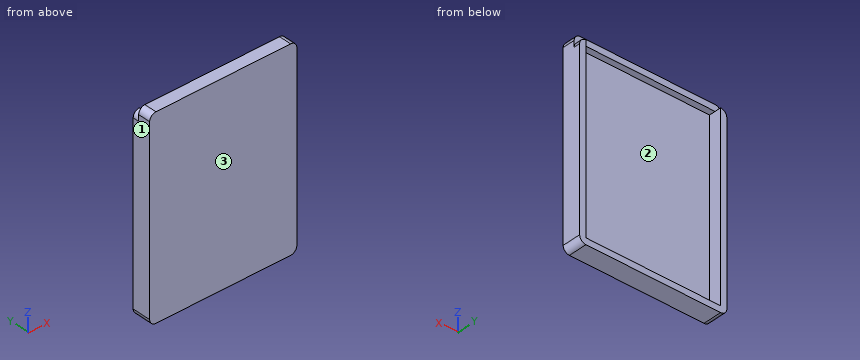
Autodesk Inventor part; units mm, degrees
ref_plane "YZ Plane" through (0, 0, 0) normal (1, 0, 0) x (0, 1, 0)
ref_plane "XZ Plane" through (0, 0, 0) normal (0, 1, 0) x (-1, 0, 0)
ref_plane "XY Plane" through (0, 0, 0) normal (0, 0, 1) x (1, 0, 0)
sketch "Sketch1" plane through (0, 0, 0) normal (0, 1, 0) x (-1, 0, 0)
  line L0 (-23.55, -31) -> (23.55, -31)
  line L1 (23.55, -31) -> (23.55, 31)
  line L2 (23.55, 31) -> (-23.55, 31)
  line L3 (-23.55, 31) -> (-23.55, -31)
  line L4 (-23.55, -31) -> (23.55, 31) construction
  line L5 (23.55, -31) -> (-23.55, 31) construction
  point P0 (0, 0)
  dimension "d0" = 47.1
  dimension "d1" = 62
extrude "Extrusion1" add sketch "Sketch1" along normal blind 2
sketch "Sketch2" plane through (0, 2, 0) normal (0, 1, 0) x (1, 0, 0)
  line L0 (-23.55, 31) -> (-23.55, -31)
  line L1 (23.55, -31) -> (23.55, 31)
  line L2 (-23.55, -31) -> (23.55, -31)
  line L3 (23.55, -31) -> (23.55, 31)
  line L4 (23.55, 31) -> (-23.55, 31)
  line L5 (-23.55, 31) -> (-23.55, -31)
  line L6 (-21.55, -29) -> (21.55, -29)
  line L7 (21.55, -29) -> (21.55, 29)
  line L8 (21.55, 29) -> (-21.55, 29)
  line L9 (-21.55, 29) -> (-21.55, -29)
  point P0 (0, 0)
  dimension "d4" = 2
  dimension "d5" = 2
  dimension "d6" = 2
  dimension "d7" = 2
extrude "Extrusion2" add sketch "Sketch2" along normal blind 2
sketch "Sketch3" plane through (0, 4, 0) normal (0, 1, 0) x (1, 0, 0)
  line L0 (-23.55, 31) -> (-23.55, -31)
  line L1 (23.55, 31) -> (-23.55, 31)
  line L2 (-23.55, 31) -> (-23.55, -29)
  line L3 (23.55, -29) -> (23.55, 31)
  line L4 (21.55, 29) -> (21.55, -29)
  line L5 (-21.55, -29) -> (-21.55, 29)
  line L6 (21.55, 29) -> (-21.55, 29)
  line L7 (-21.55, 29) -> (-21.55, -29)
  line L8 (-21.55, -29) -> (21.55, -29)
  line L9 (21.55, -29) -> (21.55, 29)
  line L10 (-21.55, -29) -> (-23.55, -29)
  line L11 (21.55, -29) -> (23.55, -29)
  line L12 (23.55, -31) -> (23.55, 31)
  line L13 (-23.55, -31) -> (23.55, -31)
  point P0 (0, 0)
extrude "Extrusion3" add sketch "Sketch3" along normal blind 2 contours L1 L3 L11 L4 L6 L5 L10 L0
fillet "Fillet1" radius 2 6 edges at (23.55, 2, 31) (23.55, 3, -31) (-23.55, 3, -31) (-23.55, 5, 29) (23.55, 5, 29) (-23.55, 2, 31)
properties part number "esp_shield_holder"
Input: part model. Units: mm. Frame: model coordinates. Face numbers are marked on the shaded views. Round coordinates to 2 decimals unless told otherwise and drop trailing zeros. Loops run counter-clockwise (first coordinate to the right, second up) from the corner with the lowest first, then second, coordinate; pieces in that order, holes last. Notation, with made-up numbers: (-21, 21.5) -> (21, 21.5) arc R19 ccw to (21, 57.5) -> close; hole circle Ø9 at (-33, -17.75). An arc over 180 degrees is marked (long way). Answer as a JSON object with one key per item and string values. Group by question number.
1) Ray query, L1, parallel to X at y = 4.5, z = -15; L2, parallel to Z at x = 19, y = 3.1; L3, parallel to Z at x = 16.5, y = 5.35. Return the intervals inside material, ascending.
2) Pin query (flat end, axial travel): pin 1 (10 mm diameter, centred on x = -9, z = 5.5, fed in from +Y); pin 2 (4.5 mm diameter, centred on x = 2.5, z = 28.5, fed in from +Y). Return the tip coordinate at first contact, or that it passes through.
3) Section query B-B on z = -12.5. Output: boundary loops of the cut face in (x, y).
4) Section query A-A on y = 2.9. Output: boundary loops of the cut face in (x, z).
5) Section query C-C on x = 17. Output: boundary loops of the cut face in (y, z), plus the area to 3 significant figures.
6) Draft query along X for the marked faces 1, 2 and 3. Return one class per face: +X half, -X half, draft (parallel to the pull), parting line (faces both ways), or undercut.
Reply:
{
 "1": {"L1": "x = -23.55 to -21.55, 21.55 to 23.55", "L2": "z = -31 to -29, 29 to 31", "L3": "z = -31 to -29"},
 "2": {"pin 1": "stops at y = 2", "pin 2": "stops at y = 4"},
 "3": {"outline": "(-23.55, 0) -> (23.55, 0) -> (23.55, 6) -> (21.55, 6) -> (21.55, 2) -> (-21.55, 2) -> (-21.55, 6) -> (-23.55, 6) -> close"},
 "4": {"outline": "(-23.55, -29) arc R2 ccw to (-21.55, -31) -> (21.55, -31) arc R2 ccw to (23.55, -29) -> (23.55, 29) arc R2 ccw to (21.55, 31) -> (-21.55, 31) arc R2 ccw to (-23.55, 29) -> close; hole (-21.55, -29) -> (21.55, -29) -> (21.55, 29) -> (-21.55, 29) -> close"},
 "5": {"outline": "(0, -31) -> (6, -31) -> (6, -29) -> (2, -29) -> (2, 29) -> (4, 29) -> (4, 31) -> (0, 31) -> close", "area": "136 mm2"},
 "6": {"face 1": "-X half", "face 2": "undercut", "face 3": "draft"}
}
